Verification items for this drawing (mm, ordinates from the low corner). A direction names the side the tool comes from. Give positions to 0.01 mm unless a question says otherwise; leave off trailing zeros. Order: outer loops, then holes, each group sorted by start corner. A loop starts at its lowest first (then second) coordinate and runs counter-clockwise, first axis right, second up.
(1) Mould release check, pull along Z, two halves, no side actions. Record for the marked faces 4, 5, 6 and 7: pulls with the +Z half, pulls with the -Z half, needs draft (parallel to the pull), parting line crosses it, or undercut.
(2) Gauge pin test, flat end, axial feed: pin 1 (19 mm diameter, centred on x = 32.84, z = 62.73, fed in from +Y). Record the tip position at first contact, or that the pin passes through.
(3) Scan lines: L1, parallel to X at y = 82, z = 74 (1 decimal); L2, parallel to X at y = 81, z = 62 (1 decimal); L3, parallel to Z at x = 29, y = 14.5. Record each from-to range of solid material in increasing order.
(4) Sectioned sample at D-D on z = 44.5. Record the cut outline in (x, y), plus the area to 3 significant figures.
(5) Sectioned sample at B-B on x = 53.5. Record the cut outline in (y, z).
(6) Access from +Z, -Z, +X, -X, +Y, -Y to the whole of each face (thin tool, end or side, straight path). Record for the marked faces 1, 2 and 3.
(7) Sectioned sample at A-A on z = 90. Record the cut outline in (x, y) (1 decimal), plus the area to 3 significant figures.
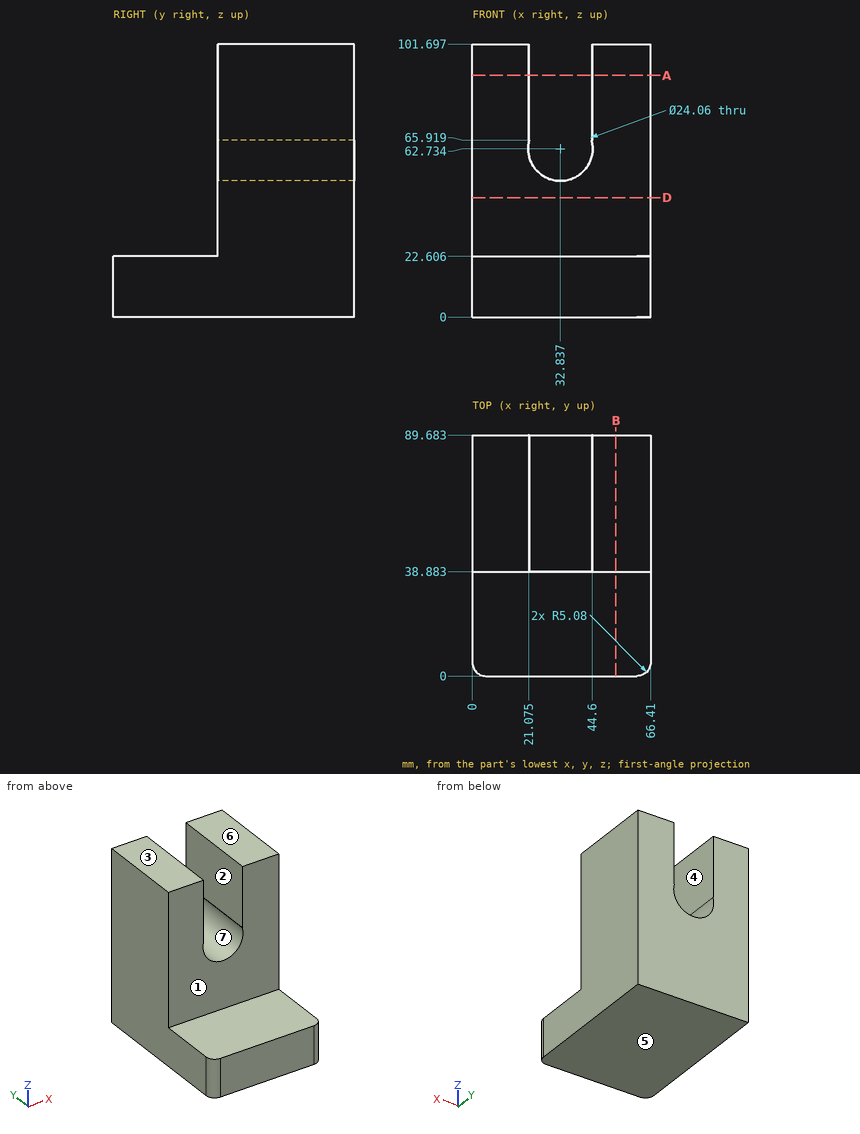
Ans:
1. face 4: needs draft
1. face 5: pulls with the -Z half
1. face 6: pulls with the +Z half
1. face 7: undercut
2. pin 1: passes through
3. L1: x = 0 to 21.1, 44.6 to 66.4
3. L2: x = 0 to 20.8, 44.8 to 66.4
3. L3: z = 0 to 22.61
4. outline: (0, 38.88) - (66.41, 38.88) - (66.41, 89.68) - (0, 89.68) - close
4. area: 3,370 mm2
5. outline: (0, 0) - (89.68, 0) - (89.68, 101.7) - (38.88, 101.7) - (38.88, 22.61) - (0, 22.61) - close
6. face 1: +Z, +X, -X, -Y
6. face 2: +Z, +Y, -Y
6. face 3: +Z, +X, -X, +Y, -Y
7. outline: (0, 38.9) - (21.1, 38.9) - (21.1, 89.7) - (0, 89.7) - close; (44.6, 38.9) - (66.4, 38.9) - (66.4, 89.7) - (44.6, 89.7) - close
7. area: 2,180 mm2
